```python
from build123d import *

# Parameters (mm, degrees)
SKETCH1_R           = 29
BOSS_EXTRUDE1_DEPTH = 3
BOSS_EXTRUDE2_DEPTH = 10
SKETCH3_R           = 29
BOSS_EXTRUDE3_DEPTH = 52
SKETCH5_R           = 2.05
CUT_EXTRUDE1_DEPTH  = 5


with BuildPart() as part:
    # Sketch1 → Boss-Extrude1 (new body)
    with BuildSketch(Plane(origin=(0, 0, 0), x_dir=(1, 0, 0), z_dir=(0, 1, 0))):
        Circle(SKETCH1_R)
    extrude(amount=BOSS_EXTRUDE1_DEPTH)

    # Sketch2 → Boss-Extrude2 (add)
    with BuildSketch(Plane(origin=(0, 3, 0), x_dir=(1, 0, 0), z_dir=(0, 1, 0))):
        with BuildLine():
            ThreePointArc((-27.349588662, 6), (-28, 0), (-27.349588662, -6))
            Line((-27.349588662, -6), (-24.784067463, -6))
            ThreePointArc((-24.784067463, -6), (-25.5, 0), (-24.784067463, 6))
            Line((-24.784067463, 6), (-27.349588662, 6))
        make_face()
        with BuildLine():
            Line((24.784067463, -6), (27.349588662, -6))
            ThreePointArc((27.349588662, -6), (27.836922267, -3.017574975), (28, 0))
            ThreePointArc((28, 0), (27.836922267, 3.017574975), (27.349588662, 6))
            Line((27.349588662, 6), (24.784067463, 6))
            ThreePointArc((24.784067463, 6), (25.320384281, 3.02128116), (25.5, 0))
            ThreePointArc((25.5, 0), (25.320384281, -3.02128116), (24.784067463, -6))
        make_face()
        with BuildLine():
            Line((-6, -24.784067463), (-6, -27.349588662))
            ThreePointArc((-6, -27.349588662), (0, -28), (6, -27.349588662))
            Line((6, -27.349588662), (6, -24.784067463))
            ThreePointArc((6, -24.784067463), (0, -25.5), (-6, -24.784067463))
        make_face()
        with BuildLine():
            ThreePointArc((6, 27.349588662), (0, 28), (-6, 27.349588662))
            Line((-6, 27.349588662), (-6, 24.784067463))
            ThreePointArc((-6, 24.784067463), (0, 25.5), (6, 24.784067463))
            Line((6, 24.784067463), (6, 27.349588662))
        make_face()
    extrude(amount=BOSS_EXTRUDE2_DEPTH)

    # Sketch3 → Boss-Extrude3 (add)
    with BuildSketch(Plane(origin=(0, 13, 0), x_dir=(1, 0, 0), z_dir=(0, 1, 0))):
        Circle(SKETCH3_R)
    extrude(amount=BOSS_EXTRUDE3_DEPTH)

    # Sketch4 → Revolve1 (revolve)
    with BuildSketch(Plane.XY):
        with BuildLine():
            Line((0, 65), (0, 72))
            ThreePointArc((0, 72), (8.804421669, 70.338678101), (16, 65))
            Line((16, 65), (0, 65))
        make_face()
    revolve(axis=Axis((0, 65, 0), (0, 1, 0)))

    # Sketch5 → Cut-Extrude1 (cut)
    with BuildSketch(Plane.XZ):
        with Locations((0, 12)):
            Circle(SKETCH5_R)
        with Locations((10.392304845, -6)):
            Circle(SKETCH5_R)
        with Locations((-10.392304845, -6)):
            Circle(SKETCH5_R)
    extrude(amount=-CUT_EXTRUDE1_DEPTH, mode=Mode.SUBTRACT)


solid = part.part
```
The listing builds one solid part. Answer for the finished solid, in the listing's coordinates (mm). A direction names the side the tool comes from. Give positions to 0.01 mm unless a question says otherwise; leave off trailing zeros. Loops run counter-clockwise (first coordinate to the right, second up) from the corner with the lowest first, then second, coordinate; pieces in that order, holes last. Notation, with made-up numbers: M 36.25,60.25 L 92.25,60.25 A11 ccw 92.25,73.25 Z; hole C 64.25,-8 d7. An arc over 180 degrees is marked long. One line per item, written item: value.
Q1. Determine the mould class of faces 1 (the face through (0, 8, -28)), 2 (the face through (13.38, 38.64, 25.73)), 3 (the face through (-25.5, 7.9, 0.1)), 4 (the face through (12, 65, 12)) for opening direction Y: +Y half, -Y half, draft (parallel to the pull), parting line (faces both ways), or undercut.
Working result:
face 1: undercut
face 2: draft
face 3: undercut
face 4: +Y half
Q2. A cutting plane is placed at B-B on z = 22. Determine the outline of the cut face in (x, y), then the cut area to 3 significant figures.
Working result:
outline: M -18.89,0 L 18.89,0 L 18.89,3 L -18.89,3 Z; M -18.89,13 L 18.89,13 L 18.89,65 L -18.89,65 Z
area: 2,080 mm^2
Q3. For faces 5 (the face through (26, 8, -6)), 6 (the face through (0.1, 7.9, 25.5)), 7 (the face through (-26, 8, 6)), determine the directions among +Z, -Z, +X, -X, +Y, -Y from which every point of the face is accessible in a straight line to the end or side of a thin tool.
Working result:
face 5: -Z, +X, -X
face 6: none
face 7: +Z, +X, -X
Q4. A cutting plane is placed at A-A on x = -17. Determine the outline of the cut face in (y, z).
Working result:
outline: M 0,-23.49 L 3,-23.49 L 3,23.49 L 0,23.49 Z; M 13,-23.49 L 65,-23.49 L 65,23.49 L 13,23.49 Z
Q5. Flat-ended cylindrical pins translate along their axes: P1, Ø1.3, axis at x = 26.5, y = 9.5, coming from the +Z side; P2, Ø3.5, axis at x = -10.39, z = -6, coming from the +Y side; P3, Ø2, axis at y = 6.5, z = 25.5, coming from the -X side. Find the tip coordinate at first contact, or state that the pin passes through.
Working result:
P1: stops at z = 6
P2: stops at y = 69.64
P3: stops at x = -6
Q6. A cutting plane is placed at C-C on y = 61. Determine the outline of the cut face in (x, z), then the cut area to 3 significant figures.
Working result:
outline: C 0,0 d58
area: 2,640 mm^2
Q7. A cutting plane is placed at D-D on z = 11. Give the number of separate pieces and of enclosed holes in the cut face, then the cut area to 3 significant figures.
Working result:
separate pieces: 3
enclosed holes: 0
area: 3,010 mm^2
Q8. Find the intervals of material crossed by line 1 (Y direction, x = 5.5, z = -21); line 2 (Y direction, x = -12.5, z = 7.5); line 3 (X direction, y = 26, z = -1), in increasing order. Write a range as from..to.
Working result:
line 1: y = 0..3, 13..65
line 2: y = 0..3, 13..66.5
line 3: x = -28.98..28.98
